from build123d import *

# Parameters (mm, degrees)
SM_BASE_FLANGE_1_DEPTH = 2.5
HOLE_WIZARD_M31_D      = 2.5
HOLE_WIZARD_M31_DEPTH  = 8.5
HOLE_WIZARD_M31_TIP    = 0.751075774
OTHER_START            = 2
OTHER_1_DEPTH          = 11
OTHER_1_2_DEPTH        = 11


# Read off the part's stored shape, not the designer's step: Нарисованный сгиб1
# Sheet-metal steps are written as plain solids
with BuildPart() as part:
    # Sketch 1 → Базовая кромка1 (new body)
    with BuildSketch(Plane.XY):
        Polygon((24, 15), (24, 13), (44, 13), (44, 2), (24, 2), (24, 0), (0, 0), (0, 15), align=None)
    extrude(amount=-SM_BASE_FLANGE_1_DEPTH)

    # Отверстие обработанное метчиком M31
    with Locations(Plane.XY):
        with Locations((3, 7.5), (15, 7.5)):
            Hole(HOLE_WIZARD_M31_D / 2, depth=HOLE_WIZARD_M31_DEPTH)
            with Locations((0, 0, -(HOLE_WIZARD_M31_DEPTH + HOLE_WIZARD_M31_TIP / 2))):  # 118° drill point
                Cone(0, HOLE_WIZARD_M31_D / 2, HOLE_WIZARD_M31_TIP, mode=Mode.SUBTRACT)

    # Other 1 outline → Other 1 (cut)
    with BuildSketch(Plane(origin=(0, 0, 0), x_dir=(1, 0, 0), z_dir=(0, 1, 0)).offset(OTHER_START)):
        with BuildLine():
            Line((44, 2.5), (29.275370017, 2.5))
            Line((29.275370017, 2.5), (26.867249414, 0.813815801))
            ThreePointArc((26.867249414, 0.813815801), (25.639331548, 0.208273722), (24.28615545, 0))
            Line((24.28615545, 0), (44, 0))
            Line((44, 0), (44, 2.5))
        make_face()
    extrude(amount=OTHER_1_DEPTH, mode=Mode.SUBTRACT)

    # Other 1 2 outline → Other 1 2 (add)
    with BuildSketch(Plane(origin=(0, 0, 0), x_dir=(1, 0, 0), z_dir=(0, 1, 0)).offset(OTHER_START)):
        with BuildLine():
            Line((29.275370017, 2.5), (42.665543077, 11.875900115))
            Line((42.665543077, 11.875900115), (41.231601986, 13.923780225))
            Line((41.231601986, 13.923780225), (25.433308323, 2.861695911))
            ThreePointArc((25.433308323, 2.861695911), (24.887567049, 2.592566099), (24.28615545, 2.5))
            Line((24.28615545, 2.5), (29.275370017, 2.5))
        make_face()
    extrude(amount=OTHER_1_2_DEPTH)


solid = part.part
Verification items for the finished model (mm, model axes). A direction names the side the tool comes from. Coordinates: 2 decimals unless noted, no trailing zeros. Order: outer loops, then holes, each group sorted by start corner. A loop starts at its lowest first (then second) coordinate and runs counter-clockwise, first axis right, second up. Notation, with made-up numbers: M -5.75,40 L 39.25,40 A18 ccw 39.25,63 Z; hole C 6.25,55.25 d5. An arc over 180 degrees is marked long. One line per item, written item: value. Start each with the question number.
Item 1: Sectioned sample at D-D (x = 3.5). Enter the section's corners in (y, z), then the cut area to 3 significant figures.
Item 2: Sectioned sample at B-B (x = 15). Enter the section's corners in (y, z), then the cut area to 4 significant figures.
Item 3: Scan lines: probe 1 along Y at (x, z) = (3, -1.75); probe 2 along Z at (x, y) = (10.5, 3.75); probe 3 along Z at (x, y) = (25, 2.25). Record each from-to range of solid material in increasing order.
Item 4: Sectioned sample at A-A (y = 7.5). Enter the section's corners in (x, z), then the cut area to 3 significant figures.
Item 5: Gauge pin test, flat ends, axial feed: pin 1 (1.5 mm diameter, centred on x = 8.5, y = 11.5, fed in from -Z); pin 2 (5 mm diameter, centred on x = 30, y = 5, fed in from -Z); pin 3 (5 mm diameter, centred on x = 33, y = 13.5, fed in from -Z). Record the tip position at first contact, or that the pin passes through.
Item 6: Mould release check, pull along Y, two halves, no side actions. Record for faces 4 (the cylindrical face through (1.845, 7.021, -1.268)), 5 (the flat face through (33, 2, -7)), 6 (the flat face through (41.959, 7.423, -12.886)), 7 (the cylindrical face through (16.25, 7.55, -1.27)): released by +Y, released by -Y, zero draft, split by the parting line, or undercut.
Item 7: Access from +Z, -Z, +X, -X, +Y, -Y to the whole of each face (thin tool, end or side, straight path). Record for faces 1 (the flat face through (12, 8, -2.5)), 2 (the flat face through (24, 14, -1)), 3 (the flat face through (24, 1, -1)).
Item 8: Sectioned sample at C-C (y = 3). Enter the section's corners in (x, z).
Conclusion:
1. outline: M 0,-2.5 L 6.35,-2.5 L 6.35,0 L 0,0 Z; M 8.65,-2.5 L 15,-2.5 L 15,0 L 8.65,0 Z
1. area: 31.8 mm^2
2. outline: M 0,-2.5 L 6.25,-2.5 L 6.25,0 L 0,0 Z; M 8.75,-2.5 L 15,-2.5 L 15,0 L 8.75,0 Z
2. area: 31.25 mm^2
3. probe 1: y = 0 to 6.25, 8.75 to 15
3. probe 2: z = -2.5 to 0
3. probe 3: z = -2.63 to -0.06
4. outline: M 0,-2.5 L 1.75,-2.5 L 1.75,0 L 0,0 Z; M 4.25,-2.5 L 13.75,-2.5 L 13.75,0 L 4.25,0 Z; M 16.25,-2.5 L 24.29,-2.5 A2 cw 25.43,-2.86 L 41.23,-13.92 L 42.67,-11.88 L 26.87,-0.81 A4.5 ccw 24.29,0 L 16.25,0 Z
4. area: 101 mm^2
5. pin 1: stops at z = -2.5
5. pin 2: stops at z = -7.81
5. pin 3: stops at z = -9.88
6. face 4: undercut
6. face 5: released by -Y
6. face 6: zero draft
6. face 7: undercut
7. face 1: -Z, -X, +Y, -Y
7. face 2: +Z, -Z, +X, +Y
7. face 3: +Z, -Z, +X, -Y
8. outline: M 0,-2.5 L 24.29,-2.5 A2 cw 25.43,-2.86 L 41.23,-13.92 L 42.67,-11.88 L 26.87,-0.81 A4.5 ccw 24.29,0 L 0,0 Z
